Geometry check sheet. Reference: the model listing, model coordinates, mm. A direction names the side the tool comes from. Give positions to 0.01 mm unless a question says otherwise; leave off trailing zeros. Order: outer loops, then holes, each group sorted by start corner. A loop starts at its lowest first (then second) coordinate and runs counter-clockwise, first axis right, second up.
```python
from build123d import *

# Parameters (mm, degrees)
MODEL_R                  = 1.500000022
MODEL_R_2                = 5.85
MODEL_W                  = 5.000000237
MODEL_H                  = 10
MODEL_H_2                = 8.000000671
RESSALTO_EXTRUS_O1_DEPTH = 5


with BuildPart() as part:
    # Model → Ressalto-extrusão1 (new body)
    with BuildSketch(Plane.XY):
        Polygon((-85.499999911, 109.000001535), (-85.499999911, 119.000001535), (-80.999999874, 119.000001535), (-80.999999874, 123.000001432), (-74.199999284, 123.000001432), (-74.199999284, 121.80000149), (-71.799999703, 121.80000149), (-71.799999703, 123.000001432), (-69.999999218, 123.000001432), (-69.999999218, 126.000001536), (-71.799999703, 126.000001536), (-71.799999703, 127.200001477), (-74.199999284, 127.200001477), (-74.199999284, 126.000001536), (-80.999999874, 126.000001536), (-80.999999874, 131.000001773), (-85.499999911, 131.000001773), (-85.499999911, 141.000001773), (7.500000924, 141.000001773), (7.500000924, 131.000001773), (3.000000887, 131.000001773), (3.000000887, 126.000001536), (-3.799999703, 126.000001536), (-3.799999703, 127.200001477), (-6.199999284, 127.200001477), (-6.199999284, 126.000001536), (-7.999999768, 126.000001536), (-7.999999768, 123.000001432), (-6.199999284, 123.000001432), (-6.199999284, 121.80000149), (-3.799999703, 121.80000149), (-3.799999703, 123.000001432), (3.000000887, 123.000001432), (3.000000887, 119.000001535), (7.500000924, 119.000001535), (7.500000924, 109.000001535), (3.000000887, 109.000001535), (3.000000887, 100.000001104), (-3.999999248, 100.000001104), (-3.999999248, 90.000001104), (3.000000887, 90.000001104), (3.000000887, 75.000001296), (7.500000924, 75.000001296), (7.500000924, 64.000001177), (3.000000887, 64.000001177), (3.000000887, 63.000001432), (3.000000887, 44.000000821), (-80.999999874, 44.000000821), (-80.999999874, 63.000001432), (-80.999999874, 64.000001177), (-85.499999911, 64.000001177), (-85.499999911, 75.000001296), (-80.999999874, 75.000001296), (-80.999999874, 90.000001104), (-73.999999739, 90.000001104), (-73.999999739, 100.000001104), (-80.999999874, 100.000001104), (-80.999999874, 109.000001535), align=None)
        with Locations((-24.000000328, 113.500001691)):
            Circle(MODEL_R, mode=Mode.SUBTRACT)
        with Locations((-24.000000328, 69.500001036)):
            Circle(MODEL_R, mode=Mode.SUBTRACT)
        with Locations((-54.000000775, 113.500001691)):
            Circle(MODEL_R, mode=Mode.SUBTRACT)
        with Locations((-54.000000775, 69.500001036)):
            Circle(MODEL_R, mode=Mode.SUBTRACT)
        with Locations((-38.999999493, 95.000001416)):
            Circle(MODEL_R_2, mode=Mode.SUBTRACT)
        with Locations((-53.999999882, 59.000001177)):
            Rectangle(MODEL_W, MODEL_H, mode=Mode.SUBTRACT)
        with Locations((-24.000000119, 80.000001296)):
            Rectangle(MODEL_W, MODEL_H, mode=Mode.SUBTRACT)
        with Locations((-53.999999882, 135.000002109)):
            Rectangle(MODEL_W, MODEL_H_2, mode=Mode.SUBTRACT)
        with Locations((-24.000000119, 135.000002109)):
            Rectangle(MODEL_W, MODEL_H_2, mode=Mode.SUBTRACT)
        with Locations((-24.000000119, 59.000001177)):
            Rectangle(MODEL_W, MODEL_H, mode=Mode.SUBTRACT)
        with Locations((-53.999999882, 80.000001296)):
            Rectangle(MODEL_W, MODEL_H, mode=Mode.SUBTRACT)
    extrude(amount=RESSALTO_EXTRUS_O1_DEPTH)


solid = part.part
```
Q1. Cross-section at B-B, the plane y = 93. Record the boundary of the cut face in (x, z).
Q2. Cross-section at A-A, the plane x = -54. Record the boundary of the cut face in (y, z), and give its area (3 significant figures).
Q3. Thickness scan on L1, parallel to Y at x = -54, z = 2.6; L2, parallel to X at y = 76, z = 2.65; L3, parallel to X at y = 136, z = 1.7. Record the ranges inside material, lowest first.
Q4. Gauge pin test, flat ends, axial feed: P1, Ø1, axis at y = 126.5, z = 2, coming from the -X side; P2, Ø0.6, axis at y = 127, z = 3, coming from the +X side. Record the tip position at first contact, or that the pin passes through.
Q5. Release check for a two-part mould opening along X. For faces 5 (the face through (-21.5, 80, 2)), 6 (the face through (-24, 64, 2)), 7 (the face through (-8, 125, 2)), 8 (the face through (5, 109, 2)) record: pulls with the +X half, pulls with the -X half, needs draft (parallel to the pull), parting line crosses it, or undercut.
Q6. Access from +Z, -Z, +X, -X, +Y, -Y to the whole of each face (thin tool, end or side, straight path). Record for faces 1 (the face through (-83, 131, 2)), 2 (the face through (-5, 127.2, 2)), 3 (the face through (0, 100, 2)), 4 (the face through (7.5, 114, 2)).
Q7. Cross-section at C-C, the plane x = -39. Record the boundary of the cut face in (y, z), and give its area (4 significant figures).
Q8. Cross-section at D-D, the plane z = 2.1. Give the number of separate pieces and of enclosed holes in the cut face, and give its area (3 significant figures).
Answers follow:
1. outline: (-74, 0) - (-44.5, 0) - (-44.5, 5) - (-74, 5) - close; (-33.5, 0) - (-4, 0) - (-4, 5) - (-33.5, 5) - close
2. outline: (44, 0) - (54, 0) - (54, 5) - (44, 5) - close; (64, 0) - (68, 0) - (68, 5) - (64, 5) - close; (71, 0) - (75, 0) - (75, 5) - (71, 5) - close; (85, 0) - (112, 0) - (112, 5) - (85, 5) - close; (115, 0) - (131, 0) - (131, 5) - (115, 5) - close; (139, 0) - (141, 0) - (141, 5) - (139, 5) - close
2. area: 315 mm2
3. L1: y = 44 to 54, 64 to 68, 71 to 75, 85 to 112, 115 to 131, 139 to 141
3. L2: x = -81 to -56.5, -51.5 to -26.5, -21.5 to 3
3. L3: x = -85.5 to -56.5, -51.5 to -26.5, -21.5 to 7.5
4. P1: stops at x = -81
4. P2: stops at x = 3
5. face 5: undercut
5. face 6: undercut
5. face 7: pulls with the +X half
5. face 8: needs draft
6. face 1: +Z, -Z, -X
6. face 2: +Z, -Z
6. face 3: +Z, -Z, +X
6. face 4: +Z, -Z, +X, +Y, -Y
7. outline: (44, 0) - (89.15, 0) - (89.15, 5) - (44, 5) - close; (100.85, 0) - (141, 0) - (141, 5) - (100.85, 5) - close
7. area: 426.5 mm2
8. separate pieces: 1
8. enclosed holes: 11
8. area: 7,790 mm2
